from build123d import *

# Parameters (mm, degrees)
SKETCH1_R           = 25
SKETCH1_R_2         = 5
SKETCH1_R_3         = 4
BOSS_EXTRUDE1_DEPTH = 9
SKETCH2_R           = 18
CUT_EXTRUDE1_DEPTH  = 4
SKETCH3_R           = 6
SKETCH3_R_2         = 4
BOSS_EXTRUDE2_DEPTH = 1
SCALE1_SCALE        = 1.5


with BuildPart() as part:
    # Sketch1 → Boss-Extrude1 (new body)
    with BuildSketch(Plane.XY):
        Circle(SKETCH1_R)
        with Locations((0, 12)):
            Circle(SKETCH1_R_2, mode=Mode.SUBTRACT)
        with Locations((12, 0)):
            Circle(SKETCH1_R_2, mode=Mode.SUBTRACT)
        with Locations((0, -12)):
            Circle(SKETCH1_R_2, mode=Mode.SUBTRACT)
        with Locations((-12, 0)):
            Circle(SKETCH1_R_2, mode=Mode.SUBTRACT)
        Circle(SKETCH1_R_3, mode=Mode.SUBTRACT)
    extrude(amount=BOSS_EXTRUDE1_DEPTH)

    # Sketch2 → Cut-Extrude1 (cut)
    with BuildSketch(Plane(origin=(0, 0, 0), x_dir=(-1, 0, 0), z_dir=(0, 0, -1))):
        Circle(SKETCH2_R)
    extrude(amount=-CUT_EXTRUDE1_DEPTH, mode=Mode.SUBTRACT)

    # Sketch3 → Boss-Extrude2 (add)
    with BuildSketch(Plane.XY.offset(9)):
        Circle(SKETCH3_R)
        with Locations(Location((0, 0, 0), (0, 0, 180))):
            Circle(SKETCH3_R_2, mode=Mode.SUBTRACT)
    extrude(amount=BOSS_EXTRUDE2_DEPTH)

    # Sketch4 → Cut-Revolve2 (revolve, cut)
    with BuildSketch(Plane(origin=(0, 0, 0), x_dir=(1, 0, 0), z_dir=(0, 1, 0))):
        Polygon((-25, 0), (0, -1.091523573), (0, 0), align=None)
    revolve(axis=Axis((0, 0, 1.091523573), (0, 0, -1)), mode=Mode.SUBTRACT)


with BuildPart() as part_1:
    # Scale1: scaled about (0, 0, 5.136545389)
    add(part.part.scale(SCALE1_SCALE).moved(Location((0, 0, -2.568272695))))


solid = part_1.part
Check sheet for the modelled part. Datum: model origin and axes. Units: mm. A direction names the side the tool comes from. Give positions to 0.01 mm unless a question says otherwise; leave off trailing zeros. Write each loop counter-clockwise with the first axis right and the second up, starting at its lowest first coordinate (ties: lowest second). Pieces come first, ordered by that corner, then holes. Notation, with made-up numbers: (-29, 8) -> (17, 8) arc R25 cw to (17, 25) -> close; hole circle Ø10 at (-2.5, -39). An arc over 180 degrees is marked (long way). Use one line per item in the form item = value. Start each with the question number.
1. Section check C-C (y = -4.5). Count the separate pieces of the cut face and the enclosed holes in it, and give its area (3 significant figures).
2. Section check A-A (z = 4.5). Record the cut outline in (x, y), and give its area (3 significant figures).
3. Go/stop test with flat-tipped pins: P1, Ø4, axis at y = 13, z = 5.5, coming from the -X side; P2, Ø9, axis at x = 0, y = 18, coming from the +Z side; P3, Ø3, axis at x = -1, z = 5.5, coming from the +Y side; P4, Ø4, axis at x = -5.5, z = 0.5, coming from the +Y side. Record where each tip stops, or that it passes through.
4. Thickness scan on line 1 along Y through (x, z) = (0, 8.5); line 2 along Y through (x, z) = (0, 1.4). Record the ranges inside material, lowest first. Write a range as from..to.
5. Access from +Z, -Z, +X, -X, +Y, -Y to the whole of each face (thin tool, end or side, straight path). Record for faces 4 (the flat face through (6.4, 0.4, 3.432)), 5 (the cylindrical face through (-0.976, 25.436, 7.129)), 6 (the flat face through (8, -8, 10.932)).
6. Mould release check, pull along X, two halves, no side actions. Record for faces 1 (the flat face through (2, -6, 12.432)), 2 (the cylindrical face through (-4.88, 37.18, 4.09)), 3 (the cylindrical face through (-0.976, -10.564, 7.129)): pulls with the +X half, pulls with the -X half, needs draft (parallel to the pull), parting line crosses it, or undercut.
7. Section check B-B (z = 0.5). Record the cut outline in (x, y).
Conclusion:
q1.separate_pieces = 4
q1.enclosed_holes = 0
q1.area = 453 mm²
q2.outline = circle Ø75 at (0, 0); hole circle Ø15 at (-18, 0); hole circle Ø15 at (0, -18); hole circle Ø15 at (0, 18); hole circle Ø12 at (0, 0); hole circle Ø15 at (18, 0)
q2.area = 3,600 mm²
q3.P1 = -35.85
q3.P2 = through
q3.P3 = 37.5
q3.P4 = 37.34
q4.line_1 = -37.5..-25.5, -10.5..-6, 6..10.5, 25.5..37.5
q4.line_2 = -37.5..-27, 27..37.5
q5.face_4 = -Z
q5.face_5 = +Z, -Z
q5.face_6 = +Z
q6.face_1 = needs draft
q6.face_2 = parting line crosses it
q6.face_3 = undercut
q7.outline = circle Ø75 at (0, 0); hole circle Ø54 at (0, 0)
